Here's how the part is built. I have some questions about the finished solid (model axes, mm). A direction names the side the tool comes from. Give positions to 0.01 mm unless a question says otherwise; leave off trailing zeros. Write each loop counter-clockwise with the first axis right and the second up, starting at its lowest first coordinate (ties: lowest second). Pieces come first, ordered by that corner, then holes. Notation, with made-up numbers: M 68.25,11 L 100.25,11 A24 ccw 100.25,41 Z; hole C 37.25,13.5 d1. An arc over 180 degrees is marked long. Answer as CSV lines item,"result". Start each with the question number.
Q1. If I drill on line 1 along Y through (x, z) = (-0.05, 4.42); line 2 along X through (y, z) = (1.25, 0); line 3 along X through (y, z) = (2.15, 3.5), over which ranges is the centre line in solid material (lowest first)?
Q2. Suppose I cut it at D-D (y = 2.2). Write out the boundary of the cut face in (x, z), then the cut area to 3 significant figures.
Q3. For pin 1 (1.5 mm diameter, centred on y = 1.5, z = 2.5, fed in from -X); pin 2 (4 mm diameter, centred on x = -5, z = 2.5, fed in from -Y); pin 3 (3 mm diameter, centred on y = 1, z = 0, fed in from -X), each with a flat end and sliding along its axis, tell me the tip position at first contact or that it passes through.
Q4. Suppose I cut it at B-B (z = 0). Write out the boundary of the cut face in (x, y).
Q5. Suppose I cut it at A-A (y = 0.3). Write out the boundary of the cut face in (x, z).
Q6. Thinking about a two-plate mould opening in X: for faces 1 (the flat face through (0, 2, 1)), 2 (the flat face through (-2, 1, -1.25)), 3 (the flat face through (-5.061, 0.183, 0.018)), 4 (the flat face through (-1.764, 2, 0)), which applies, +X half, -X half, draft (parallel to the pull), parting line (faces both ways), or undercut?
Q7. On a 3-axis mill with a long thin cutter (end or side, diameter ignored), from which of +Z, -Z, +X, -X, +Y, -Y can I reach the whole of each face in a straight line? I mean faces 5 (the flat face through (-2.164, 2, 0)), 6 (the flat face through (-5.27, -0.166, 0.018)), 7 (the flat face through (-0.4, 2, 1)). Say none if no direction works.
Q8. Suppose I cut it at C-C (y = 2.95). Write out the boundary of the cut face in (x, z).
```python
from build123d import *

# Parameters (mm, degrees)
BOSS_EXTRUDE1_DEPTH = 1.25
SKETCH2_W           = 0.4
SKETCH2_H           = 3.619533261
BOSS_EXTRUDE2_DEPTH = 4.5
SKETCH3_W           = 4
SKETCH3_H           = 1
CUT_EXTRUDE1_DEPTH  = 4.5
SKETCH4_R           = 0.25
CUT_EXTRUDE2_DEPTH  = 4.5
FILLET1_RADIUS      = 1.309766631
FILLET1_LENGTH      = 0.4


with BuildPart() as part:
    # Sketch1 → Boss-Extrude1 (new, symmetric)
    with BuildSketch(Plane.XY):
        with BuildLine():
            Line((0, 0), (0, 3.67))
            ThreePointArc((0, 3.67), (-1.08183729, 4.531548642), (-2.163674581, 3.67))
            Line((-2.163674581, 3.67), (-2.163674581, -0.5))
            ThreePointArc((-2.163674581, -0.5), (-2.274544707, -0.712979532), (-2.512599818, -0.744320081))
            Line((-2.512599818, -0.744320081), (-7.680909232, 1.136790707))
            Line((-7.680909232, 1.136790707), (-7.817717289, 0.760913659))
            Line((-7.817717289, 0.760913659), (-2.649407875, -1.12019713))
            ThreePointArc((-2.649407875, -1.12019713), (-2.045114133, -1.040640349), (-1.763674581, -0.5))
            Line((-1.763674581, -0.5), (-1.763674581, 3.619533261))
            ThreePointArc((-1.763674581, 3.619533261), (-1.08183729, 4.131548642), (-0.4, 3.619533261))
            Line((-0.4, 3.619533261), (-0.4, 0))
            Line((-0.4, 0), (0, 0))
        make_face()
    extrude(amount=BOSS_EXTRUDE1_DEPTH, both=True)

    # Sketch2 → Boss-Extrude2 (add)
    with BuildSketch(Plane.XY.offset(1.25)):
        with Locations((-0.2, 1.809766631)):
            Rectangle(SKETCH2_W, SKETCH2_H)
    extrude(amount=BOSS_EXTRUDE2_DEPTH)

    # Sketch3 → Cut-Extrude1 (cut)
    with BuildSketch(Plane(origin=(0, 0, 0), x_dir=(0, 0, -1), z_dir=(1, 0, 0))):
        with Locations((-3.75, 0.5)):
            Rectangle(SKETCH3_W, SKETCH3_H)
    extrude(amount=-CUT_EXTRUDE1_DEPTH, mode=Mode.SUBTRACT)

    # Sketch4 → Cut-Extrude2 (cut)
    with BuildSketch(Plane(origin=(0, 0, 0), x_dir=(0, 0, -1), z_dir=(1, 0, 0))):
        with Locations((-4.42, 2.309766631)):
            Circle(SKETCH4_R)
    extrude(amount=-CUT_EXTRUDE2_DEPTH, mode=Mode.SUBTRACT)

    # Fillet1: full round fillet: the end face becomes a half cylinder, R = half its width
    fillet1_face = Plane((-0.2, 2.309766631, 5.75), x_dir=(-1, 0, 0), z_dir=(0, 0, 1))  # on the end face: x along it, z out of the body
    fillet1_slab = fillet1_face.offset(-FILLET1_RADIUS / 2) * Box(FILLET1_LENGTH, 2 * FILLET1_RADIUS, FILLET1_RADIUS, mode=Mode.PRIVATE)  # the body's end, R deep
    fillet1_round = Plane((-0.2, 2.309766631, 4.440233369), x_dir=(0, 0, 1), z_dir=(-1, 0, 0)) * Cylinder(FILLET1_RADIUS, FILLET1_LENGTH, mode=Mode.PRIVATE)  # its axis R under the face
    add(fillet1_slab - fillet1_round, mode=Mode.SUBTRACT)


solid = part.part
```
Resolved:
1,line 1,"1 to 2.06, 2.56 to 3.62"
1,line 2,"-2.16 to -1.76, -0.4 to 0"
1,line 3,"-0.4 to 0"
2,outline,"M -2.16,-1.25 L -1.76,-1.25 L -1.76,1.25 L -2.16,1.25 Z; M -0.4,-1.25 L 0,-1.25 L 0,4.2 L -0.4,4.2 Z; M -0.4,4.64 L 0,4.64 L 0,5.75 L -0.4,5.75 Z"
2,area,"3.62 mm^2"
3,pin 1,"x = -0.4"
3,pin 2,"y = -0.83"
3,pin 3,"x = -7.82"
4,outline,"M -7.82,0.76 L -2.65,-1.12 A0.66 ccw -1.76,-0.5 L -1.76,3.62 A0.71 cw -0.4,3.62 L -0.4,0 L 0,0 L 0,3.67 A1.11 ccw -2.16,3.67 L -2.16,-0.5 A0.26 cw -2.51,-0.74 L -7.68,1.14 Z"
5,outline,"M -6.55,-1.25 L -5.38,-1.25 L -5.38,1.25 L -6.55,1.25 Z; M -2.16,-1.25 L -1.76,-1.25 L -1.76,1.25 L -2.16,1.25 Z; M -0.4,-1.25 L 0,-1.25 L 0,1.75 L -0.4,1.75 Z"
6,face 1,"+X half"
6,face 2,"draft"
6,face 3,"undercut"
6,face 4,"undercut"
7,face 5,"+Z, -Z, +Y"
7,face 6,"+Z, -Z, -X, -Y"
7,face 7,"+Z, -Z, -Y"
8,outline,"M -2.16,-1.25 L -1.76,-1.25 L -1.76,1.25 L -2.16,1.25 Z; M -0.4,-1.25 L 0,-1.25 L 0,5.58 L -0.4,5.58 Z"
